from build123d import *

# Parameters (mm, degrees)
BOSS_EXTRUDE1_DEPTH = 1.5
SKETCH2_R           = 1.5
CUT_EXTRUDE1_DEPTH  = 108.510464607
FILLET1_R           = 3
SKETCH8_R           = 2.5
CUT_EXTRUDE2_DEPTH  = 107.126175316
SKETCH9_R           = 1.5
CUT_EXTRUDE3_DEPTH  = 107.126175316


with BuildPart() as part:
    # Sketch1 → Boss-Extrude1 (new body)
    with BuildSketch(Plane(origin=(0, 0, 0), x_dir=(1, 0, 0), z_dir=(0, 1, 0))):
        with BuildLine():
            Line((76.013978978, 8.838834765), (58.336309448, -8.838834765))
            ThreePointArc((58.336309448, -8.838834765), (33.587572106, 0), (8.838834765, -8.838834765))
            Line((8.838834765, -8.838834765), (-8.838834765, 8.838834765))
            ThreePointArc((-8.838834765, 8.838834765), (0, 33.587572106), (-8.838834765, 58.336309448))
            Line((-8.838834765, 58.336309448), (8.838834765, 76.013978978))
            ThreePointArc((8.838834765, 76.013978978), (33.587572106, 67.175144213), (58.336309448, 76.013978978))
            Line((58.336309448, 76.013978978), (76.013978978, 58.336309448))
            ThreePointArc((76.013978978, 58.336309448), (67.175144213, 33.587572106), (76.013978978, 8.838834765))
        make_face()
    extrude(amount=BOSS_EXTRUDE1_DEPTH)

    # Sketch2 → Cut-Extrude1 (cut, through all)
    with BuildSketch(Plane(origin=(0, 1.5, 0), x_dir=(1, 0, 0), z_dir=(0, 1, 0))):
        with Locations(Location((57.629202667, 68.235804385, 0), (0, 0, 270))):
            Circle(SKETCH2_R)
        with Locations(Location((68.235804385, 57.629202667, 0), (0, 0, 270))):
            Circle(SKETCH2_R)
        with Locations(Location((68.235804385, 9.545941546, 0), (0, 0, 270))):
            Circle(SKETCH2_R)
        with Locations(Location((57.629202667, -1.060660172, 0), (0, 0, 270))):
            Circle(SKETCH2_R)
        with Locations(Location((9.545941546, -1.060660172, 0), (0, 0, 270))):
            Circle(SKETCH2_R)
        with Locations(Location((-1.060660172, 9.545941546, 0), (0, 0, 270))):
            Circle(SKETCH2_R)
        with Locations(Location((-1.060660172, 57.629202667, 0), (0, 0, 270))):
            Circle(SKETCH2_R)
        with Locations(Location((9.545941546, 68.235804385, 0), (0, 0, 270))):
            Circle(SKETCH2_R)
    extrude(amount=-CUT_EXTRUDE1_DEPTH, mode=Mode.SUBTRACT)

    # Fillet1
    fillet1_edges = [part.edges().sort_by_distance(p)[0] for p in [
        (76.013978978, 0.75, -8.838834765),
        (58.336309448, 0.75, 8.838834765),
        (8.838834765, 0.75, 8.838834765),
        (-8.838834765, 0.75, -8.838834765),
        (-8.838834765, 0.75, -58.336309448),
        (8.838834765, 0.75, -76.013978978),
        (58.336309448, 0.75, -76.013978978),
        (76.013978978, 0.75, -58.336309448),
    ]]
    fillet(fillet1_edges, radius=FILLET1_R)

    # Sketch8 → Cut-Extrude2 (cut, through all)
    with BuildSketch(Plane(origin=(0, 1.5, 0), x_dir=(1, 0, 0), z_dir=(0, 1, 0))):
        with Locations(Location((33.587572106, 33.587572106, 0), (0, 0, 270))):
            Circle(SKETCH8_R)
        with Locations(Location((41.587572106, 33.587572106, 0), (0, 0, 270))):
            Circle(SKETCH8_R)
        with Locations(Location((49.587572106, 33.587572106, 0), (0, 0, 270))):
            Circle(SKETCH8_R)
        with Locations(Location((41.587572106, 41.587572106, 0), (0, 0, 270))):
            Circle(SKETCH8_R)
        with Locations(Location((49.587572106, 41.587572106, 0), (0, 0, 270))):
            Circle(SKETCH8_R)
        with Locations(Location((41.587572106, 49.587572106, 0), (0, 0, 270))):
            Circle(SKETCH8_R)
        with Locations(Location((33.587572106, 41.587572106, 0), (0, 0, 270))):
            Circle(SKETCH8_R)
        with Locations(Location((33.587572106, 49.587572106, 0), (0, 0, 270))):
            Circle(SKETCH8_R)
        with Locations(Location((17.587572106, 41.587572106, 0), (0, 0, 90))):
            Circle(SKETCH8_R)
        with Locations(Location((17.587572106, 33.587572106, 0), (0, 0, 90))):
            Circle(SKETCH8_R)
        with Locations(Location((25.587572106, 33.587572106, 0), (0, 0, 90))):
            Circle(SKETCH8_R)
        with Locations(Location((25.587572106, 49.587572106, 0), (0, 0, 90))):
            Circle(SKETCH8_R)
        with Locations(Location((25.587572106, 41.587572106, 0), (0, 0, 90))):
            Circle(SKETCH8_R)
        with Locations(Location((49.587572106, 25.587572106, 0), (0, 0, 90))):
            Circle(SKETCH8_R)
        with Locations(Location((41.587572106, 17.587572106, 0), (0, 0, 90))):
            Circle(SKETCH8_R)
        with Locations(Location((41.587572106, 25.587572106, 0), (0, 0, 90))):
            Circle(SKETCH8_R)
        with Locations(Location((17.587572106, 25.587572106, 0), (0, 0, 270))):
            Circle(SKETCH8_R)
        with Locations(Location((25.587572106, 25.587572106, 0), (0, 0, 270))):
            Circle(SKETCH8_R)
        with Locations(Location((33.587572106, 25.587572106, 0), (0, 0, 90))):
            Circle(SKETCH8_R)
        with Locations(Location((33.587572106, 17.587572106, 0), (0, 0, 90))):
            Circle(SKETCH8_R)
        with Locations(Location((25.587572106, 17.587572106, 0), (0, 0, 270))):
            Circle(SKETCH8_R)
        with BuildLine():
            Line((8.485281374, 54.447222151), (12.727922061, 58.689862838))
            ThreePointArc((12.727922061, 58.689862838), (14.495689014, 58.689862838), (14.495689014, 56.922095886))
            Line((14.495689014, 56.922095886), (10.253048327, 52.679455198))
            ThreePointArc((10.253048327, 52.679455198), (8.485281374, 52.679455198), (8.485281374, 54.447222151))
        make_face()
        with BuildLine():
            Line((54.447222151, 58.689862838), (58.689862838, 54.447222151))
            ThreePointArc((58.689862838, 54.447222151), (58.689862838, 52.679455198), (56.922095886, 52.679455198))
            Line((56.922095886, 52.679455198), (52.679455198, 56.922095886))
            ThreePointArc((52.679455198, 56.922095886), (52.679455198, 58.689862838), (54.447222151, 58.689862838))
        make_face()
        with BuildLine():
            Line((58.689862838, 12.727922061), (54.447222151, 8.485281374))
            ThreePointArc((54.447222151, 8.485281374), (52.679455198, 8.485281374), (52.679455198, 10.253048327))
            Line((52.679455198, 10.253048327), (56.922095886, 14.495689014))
            ThreePointArc((56.922095886, 14.495689014), (58.689862838, 14.495689014), (58.689862838, 12.727922061))
        make_face()
        with BuildLine():
            Line((12.727922061, 8.485281374), (8.485281374, 12.727922061))
            ThreePointArc((8.485281374, 12.727922061), (8.485281374, 14.495689014), (10.253048327, 14.495689014))
            Line((10.253048327, 14.495689014), (14.495689014, 10.253048327))
            ThreePointArc((14.495689014, 10.253048327), (14.495689014, 8.485281374), (12.727922061, 8.485281374))
        make_face()
    extrude(amount=-CUT_EXTRUDE2_DEPTH, mode=Mode.SUBTRACT)

    # Sketch9 → Cut-Extrude3 (cut, through all)
    with BuildSketch(Plane(origin=(0, 1.5, 0), x_dir=(1, 0, 0), z_dir=(0, 1, 0))):
        with Locations(Location((33.587572106, 59.587572106, 0), (0, 0, 270))):
            Circle(SKETCH9_R)
        with Locations(Location((59.587572106, 33.587572106, 0), (0, 0, 270))):
            Circle(SKETCH9_R)
        with Locations(Location((33.587572106, 7.587572106, 0), (0, 0, 270))):
            Circle(SKETCH9_R)
        with Locations(Location((7.587572106, 33.587572106, 0), (0, 0, 270))):
            Circle(SKETCH9_R)
    extrude(amount=-CUT_EXTRUDE3_DEPTH, mode=Mode.SUBTRACT)


solid = part.part
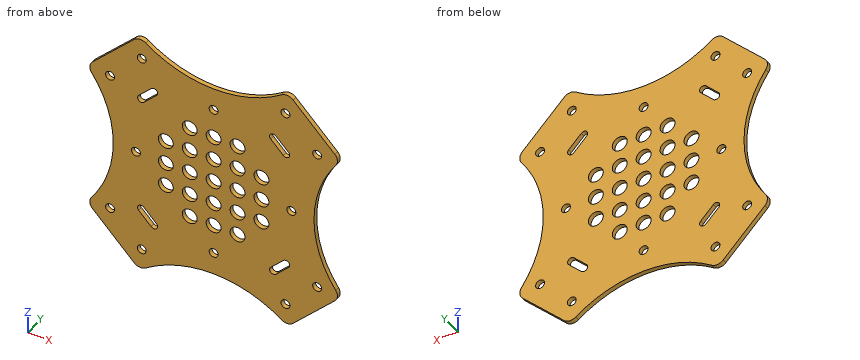
Geometry: final body of the model. Coordinates: model frame, mm. Coordinates: 2 decimals unless noted, no trailing zeros. Order: outer loops, then holes, each group sorted by start corner. A loop starts at its lowest first (then second) coordinate and runs counter-clockwise, first axis right, second up. Notation, with made-up numbers: M -38,43 L -27,43 A27 cw -27,59 Z; hole C -39.75,-35 d11. An arc over 180 degrees is marked long. One line per question, with ' | ' between items. Start each with the question number.
Item 1: Cut plane A-A, the plane z = -19. Return the cut outline in (x, y).
Item 2: Cut plane B-B, the plane y = 0.75. Count the separate pieces of the cut face and the enclosed holes in it, then the cut area to 3 significant figures.
Item 3: Ray query, probe 1 along Z at (x, y) = (41, 0.65); probe 2 along X at (y, z) = (0.8, -25); probe 3 along Z at (x, y) = (56, 0.3). Return the intervals inside material, ascending. Write a range as [from, to].
Item 4: Cut plane C-C, the plane z = -65. Return the cut outline in (x, y).
A:
1) outline: M -2.83,0 L 23.52,0 L 23.52,1.5 L -2.83,1.5 Z; M 27.65,0 L 31.52,0 L 31.52,1.5 L 27.65,1.5 Z; M 35.65,0 L 39.52,0 L 39.52,1.5 L 35.65,1.5 Z; M 43.65,0 L 70,0 L 70,1.5 L 43.65,1.5 Z
2) separate pieces: 1 | enclosed holes: 37 | area: 4,790 mm2
3) probe 1: z = [-67.88, -52.02], [-47.16, -44.02], [-39.16, -36.02], [-31.16, -28.02], [-23.16, -20.02], [-15.16, 0.71] | probe 2: x = [-0.96, 15.16], [20.02, 23.16], [28.02, 31.16], [36.02, 39.16], [44.02, 47.16], [52.02, 68.13] | probe 3: z = [-74.24, -57.14], [-53.6, -13.57], [-10.04, 7.07]
4) outline: M -2.18,0 L 69.35,0 L 69.35,1.5 L -2.18,1.5 Z
